For this review, take the finished solid that the model builds, in its own axes (mm). A direction names the side the tool comes from. Coordinates: 2 decimals unless noted, no trailing zeros. Order: outer loops, then holes, each group sorted by start corner. A loop starts at its lowest first (then second) coordinate and runs counter-clockwise, first axis right, second up. Notation, with made-up numbers: (66, -30) -> (91, -30) arc R20 cw to (91, -19) -> close; hole circle Ø9 at (82.25, 60). An arc over 180 degrees is marked (long way). Return JSON: item names as keys, results as strings. Group by question number.
Item 1: Insertion check: pin 1 (4 mm diameter, centred on y = -150, z = 106, fed in from +X); pin 2 (6.5 mm diameter, centred on x = -69.5, z = 94.5, fed in from -Y); pin 3 (3 mm diameter, centred on x = -23.5, y = 91, fed in from -Z). Each pin has a flat end and moves straight along its axis. Give the tip position at first contact, or say it passes through.
Item 2: Take a section at C-C (y = 120.5). Write out the cut boundary in (x, z), then the cut area to 3 significant figures.
Item 3: Take a section at A-A (z = 112). Write out the cut boundary in (x, y), then the cut area to 3 significant figures.
Item 4: Machinability: for faces 1 (the cylindrical face through (-4.336, -19.524, 86.465)), 2 (the flat face through (-1, 147, 106)), 3 (the flat face through (-63, -142, 128)), 4 (the flat face through (63, 142, 128)), 5 (the flat face through (67, 2, 107)), which of the approach directions +Z, -Z, +X, -X, +Y, -Y give a long, thin tool a straight path to every point of the face, cutting with its end or side? Answer none if there is none.
Item 5: Take a section at B-B (x = 26). Write out the cut boundary in (y, z), then the cut area to 3 significant figures.
Item 6: For line 1 along Y through (x, z) = (-18.5, 130.25); line 2 along Y through (x, z) = (37, 130); line 3 along Y through (x, z) = (0, 126.75), list the stretches that pass through material, from the lowest coordinate up.
Item 7: Draft analysis for pull direction Y (two halves, no side actions). For faces 6 (the flat face through (-75, 2, 108)), 7 (the cylindrical face through (-2.601, -111.715, 127.944)), 8 (the flat face through (-1, -155, 108)), state which applies: +Y half, -Y half, draft (parallel to the pull), parting line (faces both ways), or undercut.
```python
from build123d import *

# Parameters (mm, degrees)
SK_TOP_PLATE_R      = 1.7
SK_TOP_PLATE_R_2    = 12
SK_TOP_PLATE_R_3    = 15
TOP_PLATE_DEPTH     = 8
SK_FRONT_WALL_W     = 40
SK_FRONT_WALL_H     = 270
FRONT_WALL_DEPTH    = 8
SK_BACK_WALL_W      = 40
SK_BACK_WALL_H      = 270
BACK_WALL_DEPTH     = 8
SK_LEFT_WALL_W      = 110
SK_LEFT_WALL_H      = 40
LEFT_WALL_DEPTH     = 8
SK_RIGHT_WALL_W     = 110
SK_RIGHT_WALL_H     = 40
RIGHT_WALL_DEPTH    = 8
SK_BOTTOM_PLATE_R   = 47
SK_BOTTOM_PLATE_R_2 = 20
BOTTOM_PLATE_DEPTH  = 5


with BuildPart() as part:
    # SK_Top_Plate → Top_Plate (new body)
    with BuildSketch(Plane.XY.offset(124)):
        Polygon((-50, -155), (50, -155), (75, -130), (75, 130), (50, 155), (-50, 155), (-75, 130), (-75, -130), align=None)
        with Locations((37, 100)):
            Circle(SK_TOP_PLATE_R, mode=Mode.SUBTRACT)
        with Locations((18.5, 132.04293994)):
            Circle(SK_TOP_PLATE_R, mode=Mode.SUBTRACT)
        with Locations((-18.5, 132.04293994)):
            Circle(SK_TOP_PLATE_R, mode=Mode.SUBTRACT)
        with Locations((-37, 100)):
            Circle(SK_TOP_PLATE_R, mode=Mode.SUBTRACT)
        with Locations((-18.5, 67.95706006)):
            Circle(SK_TOP_PLATE_R, mode=Mode.SUBTRACT)
        with Locations((18.5, 67.95706006)):
            Circle(SK_TOP_PLATE_R, mode=Mode.SUBTRACT)
        with Locations((0, 100)):
            Circle(SK_TOP_PLATE_R_2, mode=Mode.SUBTRACT)
        with Locations((37, -100)):
            Circle(SK_TOP_PLATE_R, mode=Mode.SUBTRACT)
        with Locations((18.5, -67.95706006)):
            Circle(SK_TOP_PLATE_R, mode=Mode.SUBTRACT)
        with Locations((-18.5, -67.95706006)):
            Circle(SK_TOP_PLATE_R, mode=Mode.SUBTRACT)
        with Locations((-37, -100)):
            Circle(SK_TOP_PLATE_R, mode=Mode.SUBTRACT)
        with Locations((-18.5, -132.04293994)):
            Circle(SK_TOP_PLATE_R, mode=Mode.SUBTRACT)
        with Locations((18.5, -132.04293994)):
            Circle(SK_TOP_PLATE_R, mode=Mode.SUBTRACT)
        with Locations((0, -100)):
            Circle(SK_TOP_PLATE_R_2, mode=Mode.SUBTRACT)
        with Locations((32.04293994, 18.5)):
            Circle(SK_TOP_PLATE_R, mode=Mode.SUBTRACT)
        with Locations((0, 37)):
            Circle(SK_TOP_PLATE_R, mode=Mode.SUBTRACT)
        with Locations((-32.04293994, 18.5)):
            Circle(SK_TOP_PLATE_R, mode=Mode.SUBTRACT)
        with Locations((-32.04293994, -18.5)):
            Circle(SK_TOP_PLATE_R, mode=Mode.SUBTRACT)
        with Locations((0, -37)):
            Circle(SK_TOP_PLATE_R, mode=Mode.SUBTRACT)
        with Locations((32.04293994, -18.5)):
            Circle(SK_TOP_PLATE_R, mode=Mode.SUBTRACT)
        Circle(SK_TOP_PLATE_R_3, mode=Mode.SUBTRACT)
    extrude(amount=TOP_PLATE_DEPTH)

    # SK_Front_Wall → Front_Wall (add)
    with BuildSketch(Plane(origin=(67, 0, 0), x_dir=(0, 0, -1), z_dir=(1, 0, 0))):
        with Locations((-104, 0)):
            Rectangle(SK_FRONT_WALL_W, SK_FRONT_WALL_H)
    extrude(amount=FRONT_WALL_DEPTH)

    # SK_Back_Wall → Back_Wall (add)
    with BuildSketch(Plane(origin=(-75, 0, 0), x_dir=(0, 0, -1), z_dir=(1, 0, 0))):
        with Locations((-104, 0)):
            Rectangle(SK_BACK_WALL_W, SK_BACK_WALL_H)
    extrude(amount=BACK_WALL_DEPTH)

    # SK_Left_Wall → Left_Wall (add)
    with BuildSketch(Plane(origin=(0, 147, 0), x_dir=(1, 0, 0), z_dir=(0, 1, 0))):
        with Locations((0, -104)):
            Rectangle(SK_LEFT_WALL_W, SK_LEFT_WALL_H)
    extrude(amount=LEFT_WALL_DEPTH)

    # SK_Right_Wall → Right_Wall (add)
    with BuildSketch(Plane(origin=(0, -155, 0), x_dir=(1, 0, 0), z_dir=(0, 1, 0))):
        with Locations((0, -104)):
            Rectangle(SK_RIGHT_WALL_W, SK_RIGHT_WALL_H)
    extrude(amount=RIGHT_WALL_DEPTH)

    # SK_Bottom_Plate → Bottom_Plate (add)
    with BuildSketch(Plane.XY.offset(84)):
        Polygon((-50, -155), (50, -155), (75, -130), (75, 130), (50, 155), (-50, 155), (-75, 130), (-75, -130), align=None)
        with Locations(Location((0, 100, 0), (0, 0, 90))):
            Circle(SK_BOTTOM_PLATE_R, mode=Mode.SUBTRACT)
        with Locations(Location((0, -100, 0), (0, 0, 270))):
            Circle(SK_BOTTOM_PLATE_R, mode=Mode.SUBTRACT)
        Circle(SK_BOTTOM_PLATE_R_2, mode=Mode.SUBTRACT)
    extrude(amount=BOTTOM_PLATE_DEPTH)


solid = part.part
```
Findings below:
{
 "1": {"pin 1": "stops at x = 55", "pin 2": "stops at y = -135", "pin 3": "stops at z = 124"},
 "2": {"outline": "(-75, 84) -> (-42.29, 84) -> (-42.29, 89) -> (-67, 89) -> (-67, 124) -> (67, 124) -> (67, 89) -> (42.29, 89) -> (42.29, 84) -> (75, 84) -> (75, 132) -> (-75, 132) -> close", "area": "2,090 mm2"},
 "3": {"outline": "(-75, -135) -> (-67, -135) -> (-67, 135) -> (-75, 135) -> close; (-55, -155) -> (55, -155) -> (55, -147) -> (-55, -147) -> close; (-55, 147) -> (55, 147) -> (55, 155) -> (-55, 155) -> close; (67, -135) -> (75, -135) -> (75, 135) -> (67, 135) -> close", "area": "6,080 mm2"},
 "4": {"face 1": "-Z", "face 2": "+X, -X", "face 3": "+Z, -X, -Y", "face 4": "+Z, +X, +Y", "face 5": "+Y, -Y"},
 "5": {"outline": "(-155, 84) -> (-139.15, 84) -> (-139.15, 89) -> (-147, 89) -> (-147, 124) -> (147, 124) -> (147, 89) -> (139.15, 89) -> (139.15, 84) -> (155, 84) -> (155, 132) -> (-155, 132) -> close; (-60.85, 84) -> (60.85, 84) -> (60.85, 89) -> (-60.85, 89) -> close", "area": "3,810 mm2"},
 "6": {"line 1": "y = -155 to -133.74, -130.34 to -69.66, -66.26 to 66.26, 69.66 to 130.34, 133.74 to 155", "line 2": "y = -155 to -101.7, -98.3 to 98.3, 101.7 to 155", "line 3": "y = -155 to -112, -88 to -38.7, -35.3 to -15, 15 to 35.3, 38.7 to 88, 112 to 155"},
 "7": {"face 6": "draft", "face 7": "undercut", "face 8": "-Y half"}
}
